from build123d import *

# Parameters (mm, degrees)
BASE_EXTRUDE_DEPTH = 30


with BuildPart() as part:
    # Sketch1 → Base-Extrude (new body, symmetric)
    with BuildSketch(Plane.XY):
        with BuildLine():
            Line((39, -13.244998), (39, 22))
            ThreePointArc((39, 22), (39.87868, 24.12132), (42, 25))
            Line((42, 25), (47, 25))
            ThreePointArc((47, 25), (49.12132, 24.12132), (50, 22))
            Line((50, 22), (50, -17.41181))
            ThreePointArc((50, -17.41181), (50.085551, -18.717071), (50.340742, -20))
            Line((50.340742, -20), (51.61865, -24.769217))
            ThreePointArc((51.61865, -24.769217), (57.051725, -31.244104), (65.50409, -31.244104))
            Line((65.50409, -31.244104), (72.645011, -27.914239))
            ThreePointArc((72.645011, -27.914239), (74.938926, -27.814084), (76.631789, -29.365307))
            Line((76.631789, -29.365307), (78.322262, -32.990538))
            ThreePointArc((78.322262, -32.990538), (78.489186, -36.81373), (75.903815, -39.635168))
            Line((75.903815, -39.635168), (-10.339274, -79.850981))
            ThreePointArc((-10.339274, -79.850981), (-16.650872, -85.386104), (-19, -93.445598))
            Line((-19, -93.445598), (-19, -99))
            ThreePointArc((-19, -99), (-19.87868, -101.12132), (-22, -102))
            Line((-22, -102), (-28, -102))
            ThreePointArc((-28, -102), (-30.12132, -101.12132), (-31, -99))
            Line((-31, -99), (-31, -87.947441))
            ThreePointArc((-31, -87.947441), (-32.022225, -80.18287), (-35.019238, -72.947441))
            Line((-35.019238, -72.947441), (-47.320508, -51.641016))
            ThreePointArc((-47.320508, -51.641016), (-49.318517, -46.817397), (-50, -41.641016))
            Line((-50, -41.641016), (-50, 22))
            ThreePointArc((-50, 22), (-49.12132, 24.12132), (-47, 25))
            Line((-47, 25), (-42, 25))
            ThreePointArc((-42, 25), (-39.87868, 24.12132), (-39, 22))
            Line((-39, 22), (-39, -13.244998))
            ThreePointArc((-39, -13.244998), (-38.748418, -16.407276), (-38, -19.489996))
            ThreePointArc((-38, -19.489996), (-23.456344, -39.400616), (0, -47))
            ThreePointArc((0, -47), (23.456344, -39.400616), (38, -19.489996))
            ThreePointArc((38, -19.489996), (38.748418, -16.407276), (39, -13.244998))
        make_face()
    extrude(amount=BASE_EXTRUDE_DEPTH, both=True)

    # Sketch4 → Udboring ø26.5/ø22.5 (revolve, cut)
    with BuildSketch(Plane.XY):
        Polygon((50, 11.25), (0, 11.25), (0, 13.25), (-50, 13.25), (-50, 0), (0, 0), (50, 0), align=None)
    revolve(axis=Axis((0, 0, 0), (1, 0, 0)), mode=Mode.SUBTRACT)


solid = part.part
Could you check a few things on this model? Use its own coordinates, in mm. A direction names the side the tool comes from. Give positions to 0.01 mm unless a question says otherwise; leave off trailing zeros. Write each loop counter-clockwise with the first axis right and the second up, starting at its lowest first coordinate (ties: lowest second). Pieces come first, ordered by that corner, then holes. Notation, with made-up numbers: (45, 1.5) -> (49, 1.5) arc R35 cw to (49, 33.5) -> close; hole circle Ø1 at (5, 65.25). An arc over 180 degrees is marked (long way). Answer as CSV lines item,"result". Start each with the question number.
(1) If we mould it in two halves opening along Z, with no side actions, what happens to faces 1 (the face through (0, -48, 30)), 2 (the face through (-44.577, 7.123, 11.172)), 3 (the face through (-50, -17, 0))? For each: +Z half, -Z half, draft (parallel to the pull), parting line (faces both ways), or undercut.
(2) If we section it at A-A, the plane y = 0: Write out the boundary of the cut face in (x, z), and give its area (3 significant figures).
(3) Please list where these lines run through material, in increasing order: line 1 (X direction, y = -6.5, z = 19); line 2 (Z direction, x = -40.75, y = 0); line 3 (Z direction, x = 47, y = 0).
(4) If we section it at C-C, the plane y = -45: Write out the boundary of the cut face in (x, z).
(5) I'm going to push flat-ended pins straight in: pin 1 Ø1.7 at (y, z) = (-95, 13.5) entering from +X; pin 2 Ø24 at (y, z) = (0, 0) entering from +X; pin 3 Ø10 at (y, z) = (-69.5, 2.5) entering from +X; pin 4 Ø6 at (x, y) = (3.5, -79.5) entering from +Z. Where does each tip first touch, or does it pass through?
(6) If we section it at D-D, the plane z = 8: Give the number of separate pieces and of enclosed holes in the cut face, and give its area (3 significant figures).
(7) Which directions (+Z, -Z, +X, -X, +Y, -Y) give clear straight access to the entire face, cutting with the end or side of a thin tool? Please do faces 4 (the face through (-31.994, -80.289, 0.42)), 5 (the face through (-19, -96, 0)), 6 (the face through (-39.9, 24.14, 0.42)).
Answer list:
1,face 1,"+Z half"
1,face 2,"undercut"
1,face 3,"draft"
2,outline,"(-50, -30) -> (-39, -30) -> (-39, -13.25) -> (-50, -13.25) -> close; (-50, 13.25) -> (-39, 13.25) -> (-39, 30) -> (-50, 30) -> close; (39, -30) -> (50, -30) -> (50, -11.25) -> (39, -11.25) -> close; (39, 11.25) -> (50, 11.25) -> (50, 30) -> (39, 30) -> close"
2,area,"781 mm^2"
3,line 1,"-50 to -39, 39 to 50"
3,line 2,"-30 to -13.25, 13.25 to 30"
3,line 3,"-30 to -11.25, 11.25 to 30"
4,outline,"(-49.72, -30) -> (-12.49, -30) -> (-12.49, 30) -> (-49.72, 30) -> close; (12.49, -30) -> (64.4, -30) -> (64.4, 30) -> (12.49, 30) -> close"
5,pin 1,"x = -19"
5,pin 2,"x = 50"
5,pin 3,"x = 22.58"
5,pin 4,"through"
6,separate pieces,"3"
6,enclosed holes,"0"
6,area,"4,650 mm^2"
7,face 4,"+Z, -Z, -X, -Y"
7,face 5,"+Z, -Z, +X, -Y"
7,face 6,"+Z, -Z, +Y"
